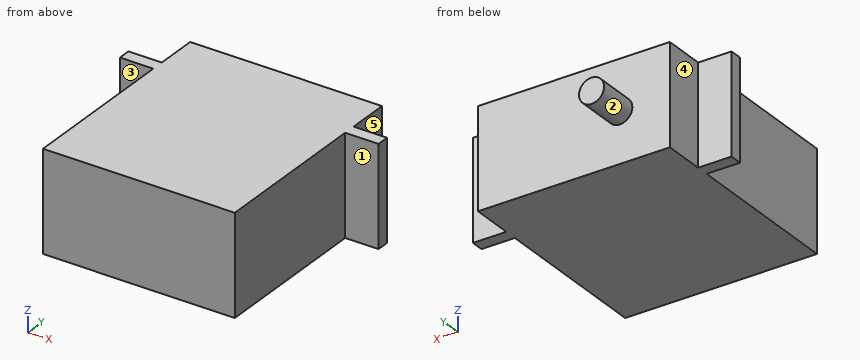
```python
from build123d import *

# Parameters (mm, degrees)
SKETCH1_W           = 23
SKETCH1_H           = 12
BOSS_EXTRUDE1_DEPTH = 26
SKETCH2_W           = 12
SKETCH2_H           = 1.5
BOSS_EXTRUDE2_DEPTH = 4
SKETCH3_R           = 1.5
BOSS_EXTRUDE3_DEPTH = 5


with BuildPart() as part:
    # Sketch1 → Boss-Extrude1 (new body)
    with BuildSketch(Plane(origin=(0, 0, 0), x_dir=(1, 0, 0), z_dir=(0, 1, 0))):
        Rectangle(SKETCH1_W, SKETCH1_H)
    extrude(amount=BOSS_EXTRUDE1_DEPTH)

    # Sketch2 → Boss-Extrude2 (add)
    with BuildSketch(Plane(origin=(11.5, 0, 0), x_dir=(0, 0, -1), z_dir=(1, 0, 0))):
        with Locations((0, 20.25)):
            Rectangle(SKETCH2_W, SKETCH2_H)
    boss_extrude2 = extrude(amount=BOSS_EXTRUDE2_DEPTH)

    # Mirror1: Boss-Extrude2 across plane
    add(boss_extrude2.mirror(Plane(origin=(0, 0, 0), x_dir=(0, 0, 1), z_dir=(1, 0, 0))))

    # Sketch3 → Boss-Extrude3 (add)
    with BuildSketch(Plane(origin=(0, 26, 0), x_dir=(1, 0, 0), z_dir=(0, 1, 0))):
        with Locations(Location((-5.5, 0, 0), (0, 0, 270))):
            Circle(SKETCH3_R)
    extrude(amount=BOSS_EXTRUDE3_DEPTH)


solid = part.part
```
For this review, take the finished solid that the model builds, in its own axes (mm). Face numbers are marked on the shaded views. A direction names the side the tool comes from. Give positions to 0.01 mm unless a question says otherwise; leave off trailing zeros. Loops run counter-clockwise (first coordinate to the right, second up) from the corner with the lowest first, then second, coordinate; pieces in that order, holes last. Notation, with made-up numbers: M -15.5,82.5 L -11.5,82.5 A12 ccw -11.5,89.5 Z; hole C -35.5,17 d11. An arc over 180 degrees is marked long. One line per item, written item: value. Start each with the question number.
Q1. For L1, parallel to X at y = 11.5, z = -4.75; L2, parallel to Y at x = -14, z = 4.5; L3, parallel to Y at x = 9.5, z = 5, list the stretches that pass through material, from the lowest coordinate up.
Q2. Machinability: for the marked faces 1, 2, 3, 4 and 5, which of the approach directions +Z, -Z, +X, -X, +Y, -Y give a long, thin tool a straight path to every point of the face, cutting with its end or side? Answer none if there is none.
Q3. Add section D-D (z = 0). Give the boundary of the cut face in (x, y), and give its area (3 significant figures).
Q4. Clearance check with flat-ended pins moving along their axes: pin 1 Ø3 at (x, z) = (-7.5, 3) entering from +Y; pin 2 Ø4 at (y, z) = (24, 0) entering from +X; pin 3 Ø3 at (x, z) = (13.5, -1.5) entering from +Y. State where each tip first meets the part, or that it passes through.
Q5. Add section B-B (z = -3.5). Give the boundary of the cut face in (x, y), and give its area (3 significant figures).
Q6. Add section A-A (x = -5.5). Give the boundary of the cut face in (y, z).
Q7. Add section C-C (y = 23). Give the boundary of the cut face in (x, z).
Reply:
1. L1: -11.5 to 11.5
1. L2: 19.5 to 21
1. L3: 0 to 26
2. face 1: +Z, -Z, +X, -Y
2. face 2: +Y
2. face 3: +Z, -Z, -X, -Y
2. face 4: +Z, -Z, -X, +Y
2. face 5: +Z, -Z, +X, +Y
3. outline: M -15.5,19.5 L -11.5,19.5 L -11.5,0 L 11.5,0 L 11.5,19.5 L 15.5,19.5 L 15.5,21 L 11.5,21 L 11.5,26 L -4,26 L -4,31 L -7,31 L -7,26 L -11.5,26 L -11.5,21 L -15.5,21 Z
3. area: 625 mm²
4. pin 1: y = 26
4. pin 2: x = 11.5
4. pin 3: y = 21
5. outline: M -15.5,19.5 L -11.5,19.5 L -11.5,0 L 11.5,0 L 11.5,19.5 L 15.5,19.5 L 15.5,21 L 11.5,21 L 11.5,26 L -11.5,26 L -11.5,21 L -15.5,21 Z
5. area: 610 mm²
6. outline: M 0,-6 L 26,-6 L 26,-1.5 L 31,-1.5 L 31,1.5 L 26,1.5 L 26,6 L 0,6 Z
7. outline: M -11.5,-6 L 11.5,-6 L 11.5,6 L -11.5,6 Z
